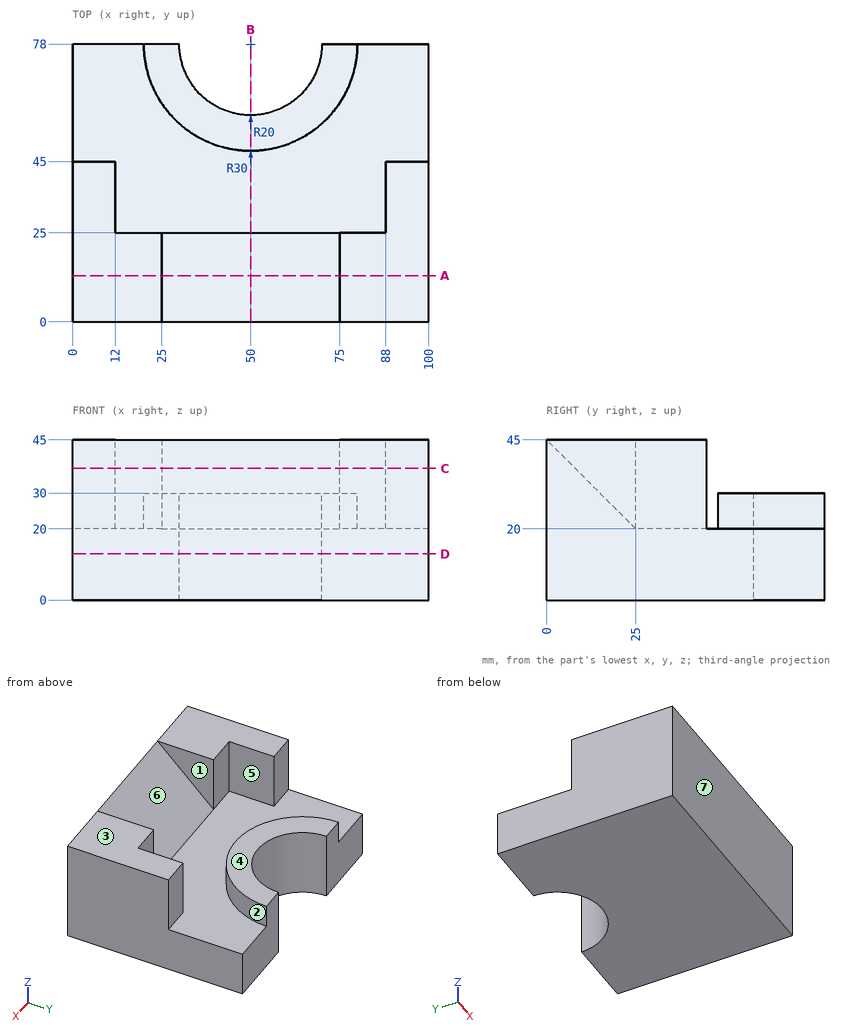
Verification items for this drawing (mm, ordinates from the low corner). A direction names the side the tool comes from. Coordinates: 2 decimals unless noted, no trailing zeros. Loops run counter-clockwise (first coordinate to the right, second up) from the corner with the lowest first, then second, coordinate; pieces in that order, holes last. Notation, with made-up numbers: (3.5, 0.25) -> (22.5, 0.25) arc R20 cw to (22.5, 5.25) -> close; hole circle Ø4 at (7.5, 36). An arc over 180 degrees is marked (long way). Answer in a Markdown table with one row per item. Add a question column.
1. Section check C-C, the plane z = 37. Enter the section's corners in (x, y), then the cut area to 3 significant figures.
2. Material ranges on probe 1 along X at (y, z) = (34.5, 36.5); probe 2 along Y at (x, z) = (14.5, 23); probe 3 along Z at (x, y) = (35, 30), recorded low to high. Write a range as [from, to].
3. Section check A-A, the plane y = 13. Enter the section's corners in (x, z).
4. Section check D-D, the plane z = 13. Enter the section's corners in (x, y).
5. Draft check along X on the marked faces 1, 2 and 3. Enter one of: +X half, -X half, draft (parallel to the pull), parting line (faces both ways), or undercut.
6. Section check B-B, the plane x = 50. Enter the section's corners in (y, z), then the cut area to 3 significant figures.
7. Depth check by flat-ended pin: P1, Ø4, axis at x = 80.5, y = 50.5, coming from the -Z side; P2, Ø10.5, axis at x = 81.5, z = 37, coming from the +Y side; P3, Ø6, axis at x = 7.5, z = 33, coming from the +Y side; P4, Ø24, axis at x = 50, y = 61.5, coming from the +Z side. Enter the tip coordinate at first touch or a pass-through.
8. Access from +Z, -Z, +X, -X, +Y, -Y to the whole of each face (thin tool, end or side, straight path). Record for the marked faces 4, 5, 6 and 7.
Derived:
| question | item | result |
|---|---|---|
| 1 | outline | (0, 0) -> (100, 0) -> (100, 45) -> (88, 45) -> (88, 25) -> (75, 25) -> (75, 8) -> (25, 8) -> (25, 25) -> (12, 25) -> (12, 45) -> (0, 45) -> close |
| 1 | area | 2,130 mm² |
| 2 | probe 1 | x = [0, 12], [88, 100] |
| 2 | probe 2 | y = [0, 25] |
| 2 | probe 3 | z = [0, 20] |
| 3 | outline | (0, 0) -> (100, 0) -> (100, 45) -> (75, 45) -> (75, 32) -> (25, 32) -> (25, 45) -> (0, 45) -> close |
| 4 | outline | (0, 0) -> (100, 0) -> (100, 78) -> (70, 78) arc R20 cw to (30, 78) -> (0, 78) -> close |
| 5 | face 1 | undercut |
| 5 | face 2 | parting line |
| 5 | face 3 | draft |
| 6 | outline | (0, 0) -> (58, 0) -> (58, 30) -> (48, 30) -> (48, 20) -> (25, 20) -> (0, 45) -> close |
| 6 | area | 1,570 mm² |
| 7 | P1 | stops at z = 0 |
| 7 | P2 | stops at y = 25 |
| 7 | P3 | stops at y = 45 |
| 7 | P4 | stops at z = 30 |
| 8 | face 4 | +Z, +X, -X, +Y |
| 8 | face 5 | +Z, +Y |
| 8 | face 6 | +Z |
| 8 | face 7 | +Z, -Z, +X, -X, -Y |
